```python
from build123d import *

# Parameters (mm, degrees)
SKETCH_1_R               = 1.75
EXTRUDE_1_DEPTH          = 27
CUT_EXTRUDE_1_DEPTH      = 33.108140695
CUT_EXTRUDE_1_DEPTH_BACK = 33.108140695
SKETCH_2_W               = 29.052061839
SKETCH_2_H               = 23


with BuildPart() as part:
    # 草图1 → 凸台-拉伸1 (new body)
    with BuildSketch(Plane(origin=(0, 0, 0), x_dir=(1, 0, 0), z_dir=(0, 1, 0))):
        with BuildLine():
            Line((-14.006965108, 3.648412425), (8.718499779, 3.648412425))
            ThreePointArc((8.718499779, 3.648412425), (10.132713341, 3.062625987), (10.718499779, 1.648412425))
            Line((10.718499779, 1.648412425), (10.718499779, -1.112487436))
            ThreePointArc((10.718499779, -1.112487436), (10.132713341, -2.526700998), (8.718499779, -3.112487436))
            Line((8.718499779, -3.112487436), (-14.006965108, -3.112487436))
            ThreePointArc((-14.006965108, -3.112487436), (-15.421178671, -2.526700998), (-16.006965108, -1.112487436))
            Line((-16.006965108, -1.112487436), (-16.006965108, 1.648412425))
            ThreePointArc((-16.006965108, 1.648412425), (-15.421178671, 3.062625987), (-14.006965108, 3.648412425))
        make_face()
        with Locations(Location((-3.445225135, 0.309187494, 0), (0, 0, 270))):
            Circle(SKETCH_1_R, mode=Mode.SUBTRACT)
        with Locations(Location((6.554774865, 0.309187494, 0), (0, 0, 270))):
            Circle(SKETCH_1_R, mode=Mode.SUBTRACT)
    extrude(amount=EXTRUDE_1_DEPTH)

    # 草图2 → 切除-拉伸1 (cut, two sides: drawn at the far end of the back side and taken through both)
    with BuildSketch(Plane.XY.offset(3.112487436).offset(-CUT_EXTRUDE_1_DEPTH_BACK)):
        with Locations((2.519065811, 13.5)):
            Rectangle(SKETCH_2_W, SKETCH_2_H)
    extrude(amount=CUT_EXTRUDE_1_DEPTH + CUT_EXTRUDE_1_DEPTH_BACK, mode=Mode.SUBTRACT)


solid = part.part
```
Here's how the part is built. I have some questions about the finished solid (model axes, mm). A direction names the side the tool comes from. Give positions to 0.01 mm unless a question says otherwise; leave off trailing zeros. Order: outer loops, then holes, each group sorted by start corner. A loop starts at its lowest first (then second) coordinate and runs counter-clockwise, first axis right, second up. Notation, with made-up numbers: M -2.5,2 L 15.5,2 A29 cw 15.5,33 Z; hole C 70.25,5.25 d2. An arc over 180 degrees is marked long. Use a Markdown table: item, result. Add a question column.
1. Suppose I cut it at D-D (x = -4.5). List the corners of the cut face in (y, z) for me, and give its area (3 significant figures).
2. Suppose I cut it at B-B (z = -1). List the corners of the cut face in (x, y) for me, and give its area (3 significant figures).
3. For pin 1 Ø2 at (y, z) = (13, 0.5) entering from +X; pin 2 Ø2 at (x, z) = (-3.45, -0.31) entering from -Y; pin 3 Ø1.5 at (y, z) = (22.5, 2.5) entering from -X, each with a flat end and sliding along its axis, tell me the tip position at first contact or that it passes through.
4. If we mould it in two halves opening along Y, with no side actions, what happens to faces 1 (the flat face through (-2, 27, -2)), 2 (the flat face through (-2, 0, -2)), 3 (the flat face through (-1, 2, 0)), 4 (the cylindrical face through (-15.41, 13.31, 2.54))? For each: +Y half, -Y half, draft (parallel to the pull), parting line (faces both ways), or undercut.
5. Suppose I cut it at A-A (x = -9.5). List the corners of the cut face in (y, z) for me.
6. I need wall thicknesses on probe 1 along Y at (x, z) = (9, -2); probe 2 along X at (y, z) = (3.5, 0); probe 3 along X at (y, z) = (14.75, 2). Which ranges of each line are inside material? Lowest first, please. Write a range as from..to.
7. On a 3-axis mill with a long thin cutter (end or side, diameter ignored), from which of +Z, -Z, +X, -X, +Y, -Y can I reach the whole of each face in a straight line? I mean faces 5 (the flat face through (-1, 25, 0)), 6 (the flat face through (10.718, 26, 0)). Say none if no direction works.
8. Suppose I cut it at C-C (y = 19.75). List the corners of the cut face in (x, z) for me.
Results list:
| question | item | result |
|---|---|---|
| 1 | outline | M 0,-3.65 L 2,-3.65 L 2,-1.71 L 0,-1.71 Z; M 0,1.09 L 2,1.09 L 2,3.11 L 0,3.11 Z; M 25,-3.65 L 27,-3.65 L 27,-1.71 L 25,-1.71 Z; M 25,1.09 L 27,1.09 L 27,3.11 L 25,3.11 Z |
| 1 | area | 15.9 mm² |
| 2 | outline | M -16.01,0 L -5.05,0 L -5.05,2 L -12.01,2 L -12.01,25 L -5.05,25 L -5.05,27 L -16.01,27 Z; M -1.84,0 L 4.95,0 L 4.95,2 L -1.84,2 Z; M -1.84,25 L 4.95,25 L 4.95,27 L -1.84,27 Z; M 8.16,0 L 10.72,0 L 10.72,2 L 8.16,2 Z; M 8.16,25 L 10.72,25 L 10.72,27 L 8.16,27 Z |
| 2 | area | 173 mm² |
| 3 | pin 1 | stops at x = -12.01 |
| 3 | pin 2 | passes through |
| 3 | pin 3 | stops at x = -15.9 |
| 4 | face 1 | +Y half |
| 4 | face 2 | -Y half |
| 4 | face 3 | undercut |
| 4 | face 4 | draft |
| 5 | outline | M 0,-3.65 L 2,-3.65 L 2,3.11 L 0,3.11 Z; M 25,-3.65 L 27,-3.65 L 27,3.11 L 25,3.11 Z |
| 6 | probe 1 | y = 0..2, 25..27 |
| 6 | probe 2 | x = -16.01..-12.01 |
| 6 | probe 3 | x = -15.8..-12.01 |
| 7 | face 5 | +Z, -Z, +X |
| 7 | face 6 | +Z, -Z, +X, +Y, -Y |
| 8 | outline | M -16.01,-1.65 A2 ccw -14.01,-3.65 L -12.01,-3.65 L -12.01,3.11 L -14.01,3.11 A2 ccw -16.01,1.11 Z |
